```python
from build123d import *

# Parameters (mm, degrees)
F0_W     = 20
F0_H     = 10
F1_DEPTH = 10
F2_W     = 14
F2_H     = 4
F3_DEPTH = 4
F5_DEPTH = 2


with BuildPart() as f1:
    # F0 (on Top) → F1 (new body)
    with BuildSketch(Plane.XY):
        Rectangle(F0_W, F0_H)
    extrude(amount=F1_DEPTH)

    # F2 (on face) → F3 (cut)
    with BuildSketch(Plane.XY.offset(10)):
        Rectangle(F2_W, F2_H)
    extrude(amount=-F3_DEPTH, mode=Mode.SUBTRACT)

    # F4 (on face) → F5 (join)
    with BuildSketch(Plane.XY.offset(6)):
        with BuildLine():
            Line((-1.5, -2), (1.5, -2))
            ThreePointArc((1.5, -2), (0, -0.4), (-1.5, -2))
        make_face()
    extrude(amount=F5_DEPTH)


solid = f1.part
```
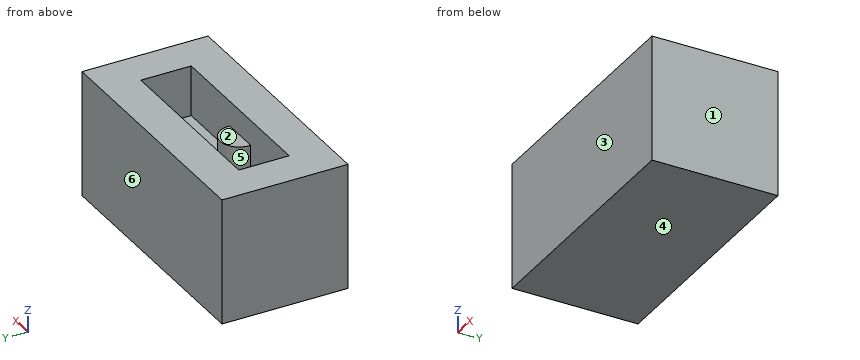
Input: part model. Units: mm. Frame: model coordinates. Face numbers are marked on the shaded views. A direction names the side the tool comes from. Give positions to 0.01 mm unless a question says otherwise; leave off trailing zeros. Order: outer loops, then holes, each group sorted by start corner. A loop starts at its lowest first (then second) coordinate and runs counter-clockwise, first axis right, second up. Notation, with made-up numbers: (-29.75, -20.5) - (4.25, -20.5) arc R23 ccw to (4.25, 10.5) - close; hole circle Ø10 at (69, 70.25). An arc over 180 degrees is marked (long way). Use a Markdown table: item, result.
(1) Section query C-C (y = 0.5). Output: boundary loops of the cut face in (x, z).
Computed values:
| item | result |
|---|---|
| outline | (-10, 0) - (10, 0) - (10, 10) - (7, 10) - (7, 6) - (-7, 6) - (-7, 10) - (-10, 10) - close |
(2) Pin query (flat end, axial travel): pin 1 (0.5 mm diameter, centred on x = 0, y = -1.5, fed in from +Z). Return the tip coordinate at first contact, or that it passes through.
Computed values:
| item | result |
|---|---|
| pin 1 | stops at z = 8 |
(3) Draft query along Y for the marked faces 3, 4, 5 and 6. Return one class per face: released by +Y, released by -Y, zero draft, split by the parting line, or undercut.
Computed values:
| item | result |
|---|---|
| face 3 | released by -Y |
| face 4 | zero draft |
| face 5 | undercut |
| face 6 | released by +Y |
(4) Line query: line 1 (X direction, y = 0.25, z = 8); line 2 (Y direction, x = -5.5, z = 6.25); line 3 (Z direction, x = 5.25, y = -1). Output: solid intervals per line, ascending. Write a range as from..to.
Computed values:
| item | result |
|---|---|
| line 1 | x = -10..-7, 7..10 |
| line 2 | y = -5..-2, 2..5 |
| line 3 | z = 0..6 |
(5) Access query for the marked faces 1 and 2. Directions: +Z, -Z, +X, -X, +Y, -Y. A direction counts if a zero-diameter tool reaches every point of the face in a straight line with its end or side. Return the directions, or none.
Computed values:
| item | result |
|---|---|
| face 1 | +Z, -Z, +X, +Y, -Y |
| face 2 | +Z |
(6) Section query D-D (x = -3.5). Output: boundary loops of the cut face in (y, z), then the cut area to 3 significant figures.
Computed values:
| item | result |
|---|---|
| outline | (-5, 0) - (5, 0) - (5, 10) - (2, 10) - (2, 6) - (-2, 6) - (-2, 10) - (-5, 10) - close |
| area | 84.0 mm2 |
(7) Section query B-B (x = 0). Output: boundary loops of the cut face in (y, z).
Computed values:
| item | result |
|---|---|
| outline | (-5, 0) - (5, 0) - (5, 10) - (2, 10) - (2, 6) - (-0.4, 6) - (-0.4, 8) - (-2, 8) - (-2, 10) - (-5, 10) - close |
(8) Section query A-A (z = 7.75). Output: boundary loops of the cut face in (x, y), then the cut area to 3 significant figures.
Computed values:
| item | result |
|---|---|
| outline | (-10, -5) - (10, -5) - (10, 5) - (-10, 5) - close; hole (-7, -2) - (-1.5, -2) arc R1.5 cw (long way) to (1.5, -2) - (7, -2) - (7, 2) - (-7, 2) - close |
| area | 148 mm2 |
